Verification items for the finished model (mm, model axes). Face numbers are marked on the shaded views. A direction names the side the tool comes from. Give positions to 0.01 mm unless a question says otherwise; leave off trailing zeros. Order: outer loops, then holes, each group sorted by start corner. A loop starts at its lowest first (then second) coordinate and runs counter-clockwise, first axis right, second up. Notation, with made-up numbers: (1.5, 51.5) -> (22.5, 51.5) arc R23 ccw to (22.5, 72.5) -> close; hole circle Ø9 at (16, 50). An arc over 180 degrees is marked (long way). Write each question's results on one line, items separated by ' | '. Start each with the question number.
1. Set-up check for the marked faces 1, 2 and 3: record each of +Z, -Z, +X, -X, +Y, -Y from which the full face is reachable in a straight line by a thin tool's end or side.
2. Depth check by flat-ended pin: pin 1 Ø6 at (y, z) = (-13.5, 31.5) entering from +X; pin 2 Ø3 at (y, z) = (10, 52) entering from +X; pin 3 Ø22 at (x, y) = (48, -13) entering from +Z. Enter the tip coordinate at first touch or a pass-through.
3. Material ranges on L1, parallel to Z at x = 24.5, y = -9; L2, parallel to X at y = 9, z = 54.5, recorded low to high. Write a range as from..to.
4. Cross-section at B-B, the plane z = 30. Enter the section's corners in (x, y), then the cut area to 3 significant figures.
5. Cross-section at A-A, the plane y = -2. Enter the section's corners in (x, z), then the cut area to 3 significant figures.
6. Cross-section at D-D, the plane z = 47.5. Enter the section's corners in (x, y).
7. Cross-section at C-C, the plane x = 53. Enter the section's corners in (y, z).
from build123d import *

# Parameters (mm, degrees)
F1_DEPTH = 20
F0_W     = 20
F0_H     = 20
F2_DEPTH = 20


with BuildPart() as f1:
    # F0 (on Front) → F1 (new body, symmetric)
    with BuildSketch(Plane.XZ):
        Polygon((0, 60), (0, 0), (60, 0), (60, 20), (40, 20), (40, 40), (20, 40), (20, 60), align=None)
    extrude(amount=F1_DEPTH, both=True)

    # F0 (on Front) → F2 (join)
    with BuildSketch(Plane.XZ):
        Polygon((0, 60), (0, 0), (60, 0), (60, 20), (40, 20), (40, 40), (20, 40), (20, 60), align=None)
        with Locations((50, 30)):
            Rectangle(F0_W, F0_H)
    extrude(amount=-F2_DEPTH)


solid = f1.part
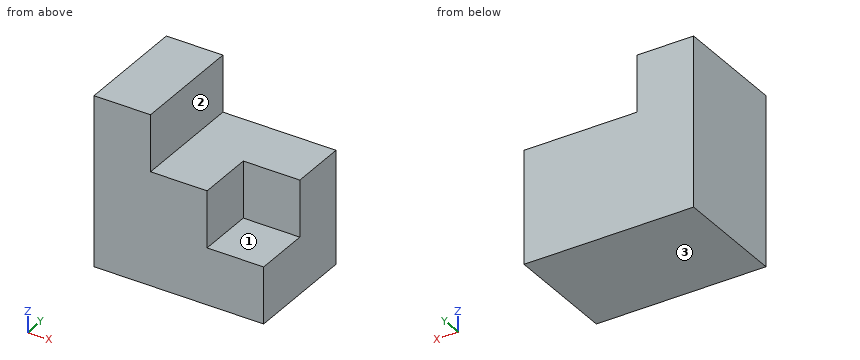
Results below:
1) face 1: +Z, +X, -Y | face 2: +Z, +X, +Y, -Y | face 3: -Z, +X, -X, +Y, -Y
2) pin 1: stops at x = 40 | pin 2: stops at x = 20 | pin 3: stops at z = 40
3) L1: z = 0..40 | L2: x = 0..20
4) outline: (0, -20) -> (40, -20) -> (40, 0) -> (60, 0) -> (60, 20) -> (0, 20) -> close | area: 2,000 mm²
5) outline: (0, 0) -> (60, 0) -> (60, 20) -> (40, 20) -> (40, 40) -> (20, 40) -> (20, 60) -> (0, 60) -> close | area: 2,400 mm²
6) outline: (0, -20) -> (20, -20) -> (20, 20) -> (0, 20) -> close
7) outline: (-20, 0) -> (20, 0) -> (20, 40) -> (0, 40) -> (0, 20) -> (-20, 20) -> close
